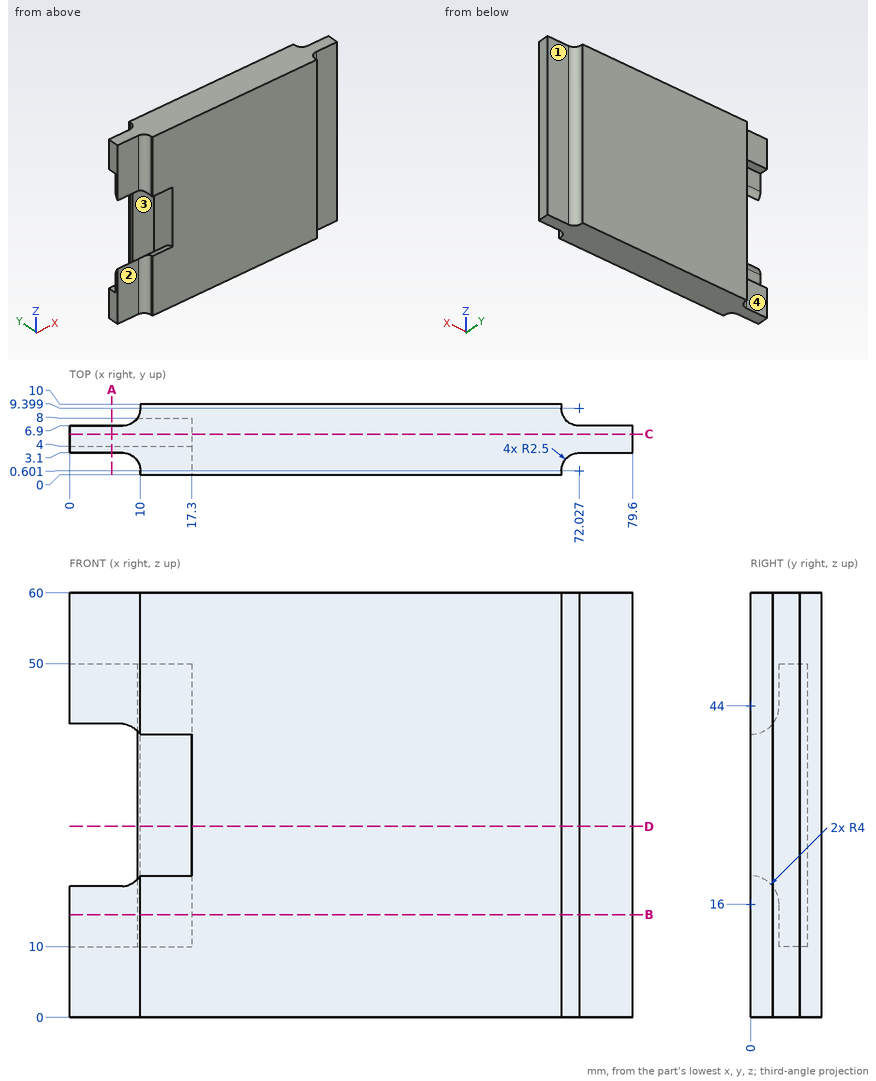
Print and shaded views of the part. All mm, measured from the part's lowest x, y and z. A direction names the side the tool comes from. Coordinates: 2 decimals unless noted, no trailing zeros. Loops run counter-clockwise (first coordinate to the right, second up) from the corner with the lowest first, then second, coordinate; pieces in that order, holes last. Notation, with made-up numbers: (-26.5, 8.25) -> (14.5, 8.25) arc R18 cw to (14.5, 24.25) -> close; hole circle Ø8 at (58.25, -34). An arc over 180 degrees is marked (long way). Use a Markdown table: item, result. Add a question column.
Item 1: Band-saw the part on C-C on y = 5.75. Write the cut outline in (x, z).
Item 2: Band-saw the part on A-A on x = 6. Write the cut outline in (y, z).
Item 3: Band-saw the part on D-D on z = 27. Write the cut outline in (x, y).
Item 4: Flat gauge pins, fed straight in: P1, Ø2, axis at y = 6, z = 17, coming from the -X side; P2, Ø8, axis at x = 4, z = 55, coming from the +Y side; P3, Ø8, axis at x = 74.5, z = 35.5, coming from the +Y side. Where does each tip first touch, or does it go through?
Item 5: Probe probe 1 along Z at (x, y) = (10.5, 2.5); probe 2 along X at (y, z) = (6.75, 17); probe 3 along X at (y, z) = (0.75, 16.5) (1 decimal). List the from-to ranges inside material, lowest first.
Item 6: Band-saw the part on B-B on z = 14.5. Write the cut outline in (x, y).
Item 7: Which spindle directions (+Z, -Z, +X, -X, +Y, -Y) get a long thin tool onto all of the face, cutting with end or side? Do the marked faces 1, 2, 3 and 4. Say none if no direction does.
Geometry says:
| question | item | result |
|---|---|---|
| 1 | outline | (0, 0) -> (79.6, 0) -> (79.6, 60) -> (0, 60) -> (0, 50) -> (17.3, 50) -> (17.3, 10) -> (0, 10) -> close |
| 2 | outline | (3.1, 0) -> (6.9, 0) -> (6.9, 10) -> (4, 10) -> (4, 16) arc R4 ccw to (3.1, 18.53) -> close; (3.1, 41.47) arc R4 ccw to (4, 44) -> (4, 50) -> (6.9, 50) -> (6.9, 60) -> (3.1, 60) -> close |
| 3 | outline | (9.57, 8) -> (17.3, 8) -> (17.3, 0) -> (69.6, 0) arc R2.5 cw to (72.1, 3.1) -> (79.6, 3.1) -> (79.6, 6.9) -> (72.1, 6.9) arc R2.5 cw to (69.6, 10) -> (10, 10) -> (10, 9.4) arc R2.5 cw to start |
| 4 | P1 | x = 17.3 |
| 4 | P2 | y = 6.95 |
| 4 | P3 | y = 7.42 |
| 5 | probe 1 | 0 to 19.12, 40.88 to 60 |
| 5 | probe 2 | 17.3 to 79.6 |
| 5 | probe 3 | 10 to 69.5 |
| 6 | outline | (0, 3.1) -> (7.5, 3.1) arc R2.5 cw to (10, 0.6) -> (10, 0) -> (69.6, 0) arc R2.5 cw to (72.1, 3.1) -> (79.6, 3.1) -> (79.6, 6.9) -> (72.1, 6.9) arc R2.5 cw to (69.6, 10) -> (10, 10) -> (10, 9.4) arc R2.5 cw to (9.57, 8) -> (17.3, 8) -> (17.3, 4) -> (0, 4) -> close |
| 7 | face 1 | +Z, -Z, +X, +Y |
| 7 | face 2 | +Z, -Z, -X, -Y |
| 7 | face 3 | -X |
| 7 | face 4 | +Z, -Z, -X, +Y |
